```python
from build123d import *

# Parameters (mm, degrees)
F0_W      = 46
F0_H      = 80
F1_DEPTH  = 1
F2_W      = 43
F2_H      = 1
F2_W_2    = 1
F2_H_2    = 77
F3_DEPTH  = 18
F4_W      = 1.5
F4_H      = 1.5
F5_DEPTH  = 1.001
F6_R      = 1.75
F7_DEPTH  = 19.001
F9_DEPTH  = 80.001
F10_W     = 11.5
F10_H     = 1
F11_DEPTH = 2
F12_W     = 1
F12_H     = 1
F13_DEPTH = 0.5
F14_R     = 1


with BuildPart() as f1:
    # F0 (on Front) → F1 (new body)
    with BuildSketch(Plane.XZ):
        Rectangle(F0_W, F0_H)
    extrude(amount=-F1_DEPTH)

    # F2 (on face) → F3 (join)
    with BuildSketch(Plane(origin=(0, 1, 0), x_dir=(-1, 0, 0), z_dir=(0, 1, 0))):
        with Locations((0, 39.5)):
            Rectangle(F2_W, F2_H)
        with Locations((-22.5, 0)):
            Rectangle(F2_W_2, F2_H_2)
        with Locations((22.5, 0)):
            Rectangle(F2_W_2, F2_H_2)
        with Locations((0, -39.5)):
            Rectangle(F2_W, F2_H)
    extrude(amount=F3_DEPTH)

    # F4 (on face) → F5 (cut, through all)
    with BuildSketch(Plane(origin=(0, 1, 0), x_dir=(-1, 0, 0), z_dir=(0, 1, 0))):
        with Locations((22.25, 39.25)):
            Rectangle(F4_W, F4_H)
        with Locations((-22.25, 39.25)):
            Rectangle(F4_W, F4_H)
        with Locations((22.25, -39.25)):
            Rectangle(F4_W, F4_H)
        with Locations((-22.25, -39.25)):
            Rectangle(F4_W, F4_H)
    extrude(amount=-F5_DEPTH, mode=Mode.SUBTRACT)

    # F6 (on face) → F7 (cut, through all)
    with BuildSketch(Plane.XZ):
        with Locations((15, -27.5)):
            Circle(F6_R)
        with Locations((-15, 27.5)):
            Circle(F6_R)
    extrude(amount=-F7_DEPTH, mode=Mode.SUBTRACT)

    # F8 (on face) → F9 (cut, through all)
    with BuildSketch(Plane.XY.offset(40)):
        with BuildLine():
            ThreePointArc((-1.5, 6.5), (0, 5), (1.5, 6.5))
            Line((1.5, 6.5), (1.5, 14.5))
            ThreePointArc((1.5, 14.5), (0, 16), (-1.5, 14.5))
            Line((-1.5, 14.5), (-1.5, 6.5))
        make_face()
        with BuildLine():
            ThreePointArc((-6.5, 6.5), (-5, 5), (-3.5, 6.5))
            Line((-3.5, 6.5), (-3.5, 14.5))
            ThreePointArc((-3.5, 14.5), (-5, 16), (-6.5, 14.5))
            Line((-6.5, 14.5), (-6.5, 6.5))
        make_face()
        with BuildLine():
            ThreePointArc((-11.5, 6.5), (-10, 5), (-8.5, 6.5))
            Line((-8.5, 6.5), (-8.5, 14.5))
            ThreePointArc((-8.5, 14.5), (-10, 16), (-11.5, 14.5))
            Line((-11.5, 14.5), (-11.5, 6.5))
        make_face()
        with BuildLine():
            ThreePointArc((-16.5, 6.5), (-15, 5), (-13.5, 6.5))
            Line((-13.5, 6.5), (-13.5, 14.5))
            ThreePointArc((-13.5, 14.5), (-15, 16), (-16.5, 14.5))
            Line((-16.5, 14.5), (-16.5, 6.5))
        make_face()
        with BuildLine():
            ThreePointArc((8.5, 6.5), (10, 5), (11.5, 6.5))
            Line((11.5, 6.5), (11.5, 14.5))
            ThreePointArc((11.5, 14.5), (10, 16), (8.5, 14.5))
            Line((8.5, 14.5), (8.5, 6.5))
        make_face()
        with BuildLine():
            ThreePointArc((3.5, 6.5), (5, 5), (6.5, 6.5))
            Line((6.5, 6.5), (6.5, 14.5))
            ThreePointArc((6.5, 14.5), (5, 16), (3.5, 14.5))
            Line((3.5, 14.5), (3.5, 6.5))
        make_face()
        with BuildLine():
            ThreePointArc((13.5, 6.5), (15, 5), (16.5, 6.5))
            Line((16.5, 6.5), (16.5, 14.5))
            ThreePointArc((16.5, 14.5), (15, 16), (13.5, 14.5))
            Line((13.5, 14.5), (13.5, 6.5))
        make_face()
    extrude(amount=-F9_DEPTH, mode=Mode.SUBTRACT)

    # F10 (on face) → F11 (join)
    with BuildSketch(Plane(origin=(0, 19, 0), x_dir=(-1, 0, 0), z_dir=(0, 1, 0))):
        with Locations((-5.75, -39.5)):
            Rectangle(F10_W, F10_H)
        with Locations((5.75, 39.5)):
            Rectangle(F10_W, F10_H)
    extrude(amount=F11_DEPTH)

    # F12 (on face) → F13 (join)
    with BuildSketch(Plane(origin=(0, 19, 0), x_dir=(-1, 0, 0), z_dir=(0, 1, 0))):
        with Locations((11.5, -39.5)):
            Rectangle(F12_W, F12_H)
        with Locations((-11.5, 39.5)):
            Rectangle(F12_W, F12_H)
        with Locations((22.5, 27.5)):
            Rectangle(F12_W, F12_H)
        with Locations((-22.5, 27.5)):
            Rectangle(F12_W, F12_H)
        with Locations((22.5, -27.5)):
            Rectangle(F12_W, F12_H)
        with Locations((-22.5, -27.5)):
            Rectangle(F12_W, F12_H)
        with Locations((22.5, 0)):
            Rectangle(F12_W, F12_H)
        with Locations((-22.5, 0)):
            Rectangle(F12_W, F12_H)
    extrude(amount=F13_DEPTH)

    # F14
    f14_edges = [f1.edges().sort_by_distance(p)[0] for p in [
        (-23, 0, 0),
        (0, 0, 40),
        (23, 0, 0),
        (0, 0, -40),
    ]]
    fillet(f14_edges, radius=F14_R)


solid = f1.part
```
CAD build for the part. Positions are in the model's coordinates, mm. A direction names the side the tool comes from. Round coordinates to 2 decimals unless told otherwise and drop trailing zeros. Write each loop counter-clockwise with the first axis right and the second up, starting at its lowest first coordinate (ties: lowest second). Pieces come first, ordered by that corner, then holes. Notation, with made-up numbers: (35.25, 33) -> (85.25, 33) arc R30 cw to (85.25, 56) -> close; hole circle Ø10 at (26.25, 30). An arc over 180 degrees is marked (long way). Answer in a Markdown table with one row per item. Add a question column.
Item 1: Mould opens along Y. For faces 5 (the face through (-5, 5, 39.5)), 6 (the face through (-14.1, 0.5, 29)), 7 (the face through (0, 5, 39.5)) say: pulls with the +Y half, pulls with the -Y half, needs draft (parallel to the pull), parting line crosses it, or undercut.
Item 2: Saw through at A-A, the plane x = 15. Write the cut outline in (y, z), then the cut area to 3 significant figures.
Item 3: Which spindle directions (+Z, -Z, +X, -X, +Y, -Y) get a long thin tool onto all of the face, cutting with end or side? Do faces 1 (the face through (0, 4, -39)), 2 (the face through (23, 10, -1)), 3 (the face through (-22.4, 9.4, -38.5)), 4 (the face through (10, 5, 39.5)). Say none if no direction does.
Item 4: Saw through at C-C, the plane z = -20.5. Write the cut outline in (x, y), then the cut area to 3 significant figures.
Item 5: Saw through at B-B, the plane x = -10. Write the cut outline in (y, z), then the cut area to 3 significant figures.
Item 6: Drop flat-ended pins along their axis: pin 1 Ø0.6 at (y, z) = (19, 39.5) entering from +X; pin 2 Ø0.5 at (x, z) = (-17.5, -39.5) entering from +Y; pin 3 Ø2 at (x, z) = (14, 7.5) entering from -Y; pin 4 Ø1.1 at (y, z) = (11, -39.5) entering from -X. Give the stop position or say it passes through.
Item 7: Drill centre lines: line 1 (Z direction, x = -11, y = 2.5); line 2 (X direction, y = 13, z = -32); line 3 (Y direction, x = 11, z = 35). Where is each one in solid material? Low to high. Write a range as from..to.
Findings below:
| question | item | result |
|---|---|---|
| 1 | face 5 | undercut |
| 1 | face 6 | needs draft |
| 1 | face 7 | undercut |
| 2 | outline | (0, -39) arc R1 ccw to (1, -40) -> (5, -40) -> (5, -39) -> (1, -39) -> (1, -29.25) -> (0, -29.25) -> close; (0, -25.75) -> (1, -25.75) -> (1, 39) -> (5, 39) -> (5, 40) -> (1, 40) arc R1 ccw to (0, 39) -> close; (16, -40) -> (19, -40) -> (19, -39) -> (16, -39) -> close; (16, 39) -> (19, 39) -> (19, 40) -> (16, 40) -> close |
| 2 | area | 90.1 mm^2 |
| 3 | face 1 | +X, -X, +Y |
| 3 | face 2 | +Z, -Z, +X, +Y, -Y |
| 3 | face 3 | -Z, -X, +Y, -Y |
| 3 | face 4 | +Z, -Z |
| 4 | outline | (-23, 1) arc R1 ccw to (-22, 0) -> (22, 0) arc R1 ccw to (23, 1) -> (23, 19) -> (22, 19) -> (22, 1) -> (-22, 1) -> (-22, 19) -> (-23, 19) -> close |
| 4 | area | 81.6 mm^2 |
| 5 | outline | (0, -39) arc R1 ccw to (1, -40) -> (5, -40) -> (5, -39) -> (1, -39) -> (1, 39) -> (5, 39) -> (5, 40) -> (1, 40) arc R1 ccw to (0, 39) -> close; (16, -40) -> (19, -40) -> (19, -39) -> (16, -39) -> close; (16, 39) -> (21, 39) -> (21, 40) -> (16, 40) -> close |
| 5 | area | 95.6 mm^2 |
| 6 | pin 1 | stops at x = 21.5 |
| 6 | pin 2 | stops at y = 19 |
| 6 | pin 3 | stops at y = 0 |
| 6 | pin 4 | stops at x = -21.5 |
| 7 | line 1 | z = -40..-39, 39..40 |
| 7 | line 2 | x = -23..-22, 22..23 |
| 7 | line 3 | y = 0..1 |
